Design review of the part built by this model. Coordinates are the model's own, in mm. Face numbers are marked on the shaded views. A direction names the side the tool comes from. Give positions to 0.01 mm unless a question says otherwise; leave off trailing zeros. Order: outer loops, then holes, each group sorted by start corner. A loop starts at its lowest first (then second) coordinate and runs counter-clockwise, first axis right, second up. Notation, with made-up numbers: M 1,60 L 22,60 A33 ccw 22,89 Z; hole C -12.75,38 d5. An arc over 180 degrees is marked long. Answer as a JSON object with one key per item and string values.
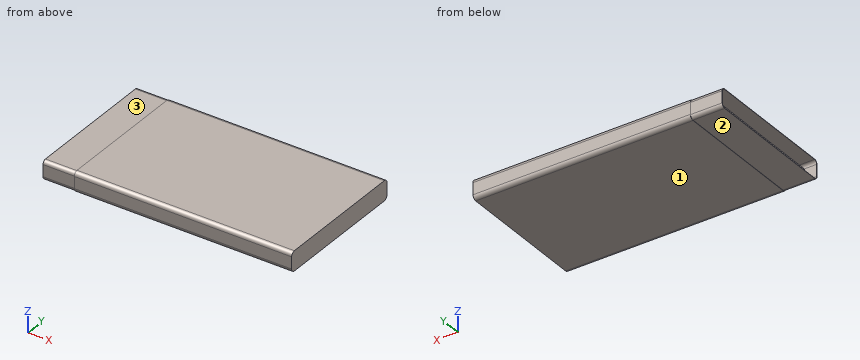
from build123d import *

# Parameters (mm, degrees)
SKETCH1_W           = 55
SKETCH1_H           = 35
BOSS_EXTRUDE1_DEPTH = 2.5
FILLET1_R           = 1
SKETCH2_W           = 5.5
SKETCH2_H           = 33
BOSS_EXTRUDE2_DEPTH = 0.8
BOSS_EXTRUDE4_DEPTH = 8


with BuildPart() as part:
    # Sketch1 → Boss-Extrude1 (new, symmetric)
    with BuildSketch(Plane.XY):
        with Locations((4, 0)):
            Rectangle(SKETCH1_W, SKETCH1_H)
    extrude(amount=BOSS_EXTRUDE1_DEPTH, both=True)

    # Fillet1
    fillet1_edges = [part.edges().sort_by_distance(p)[0] for p in [
        (4, 17.5, 2.5),
        (4, -17.5, 2.5),
        (4, 17.5, -2.5),
        (4, -17.5, -2.5),
    ]]
    fillet(fillet1_edges, radius=FILLET1_R)

    # Sketch2 → Boss-Extrude2 (add, symmetric)
    with BuildSketch(Plane.XY):
        with Locations((-26.25, 0)):
            Rectangle(SKETCH2_W, SKETCH2_H)
    extrude(amount=BOSS_EXTRUDE2_DEPTH, both=True)

    # Sketch3 → Boss-Extrude4 (add)
    with BuildSketch(Plane.ZY.offset(23.5)):
        with BuildLine():
            Line((-1.5, -17.4), (1.5, -17.4))
            ThreePointArc((1.5, -17.4), (2.136396103, -17.136396103), (2.4, -16.5))
            Line((2.4, -16.5), (2.4, 16.5))
            ThreePointArc((2.4, 16.5), (2.136396103, 17.136396103), (1.5, 17.4))
            Line((1.5, 17.4), (-1.5, 17.4))
            ThreePointArc((-1.5, 17.4), (-2.136396103, 17.136396103), (-2.4, 16.5))
            Line((-2.4, 16.5), (-2.4, -16.5))
            ThreePointArc((-2.4, -16.5), (-2.136396103, -17.136396103), (-1.5, -17.4))
        make_face()
        with BuildLine():
            Line((-1.5, -17.3), (1.5, -17.3))
            ThreePointArc((1.5, -17.3), (2.065685425, -17.065685425), (2.3, -16.5))
            Line((2.3, -16.5), (2.3, 16.5))
            ThreePointArc((2.3, 16.5), (2.065685425, 17.065685425), (1.5, 17.3))
            Line((1.5, 17.3), (-1.5, 17.3))
            ThreePointArc((-1.5, 17.3), (-2.065685425, 17.065685425), (-2.3, 16.5))
            Line((-2.3, 16.5), (-2.3, -16.5))
            ThreePointArc((-2.3, -16.5), (-2.065685425, -17.065685425), (-1.5, -17.3))
        make_face(mode=Mode.SUBTRACT)
    extrude(amount=BOSS_EXTRUDE4_DEPTH)


solid = part.part
(1) We need section B-B (y = 11). Write out the cut boundary in (x, z), plus the area to 3 significant figures.
Checked values:
{"outline": "M -31.5,-2.4 L -23.5,-2.4 L -23.5,-2.5 L 31.5,-2.5 L 31.5,2.5 L -23.5,2.5 L -23.5,2.4 L -31.5,2.4 L -31.5,2.3 L -23.5,2.3 L -23.5,0.8 L -29,0.8 L -29,-0.8 L -23.5,-0.8 L -23.5,-2.3 L -31.5,-2.3 Z", "area": "285 mm^2"}
(2) To check wall thickness, follow L1, parallel to Y at x = 18.5, z = -1.55; L2, parallel to X at y = 8.5, z = 0.7; L3, parallel to X at y = 3.5, z = -1.55. State the ranges of each line that lie inside material, in increasing order. Write a range as from..to.
Checked values:
{"L1": "y = -17.5..17.5", "L2": "x = -29..31.5", "L3": "x = -23.5..31.5"}
(3) Insertion check: pin 1 (1.6 mm diameter, centred on x = -25.5, y = -5.5, fed in from -Z); pin 2 (1.8 mm diameter, centred on y = 2.5, z = 0, fed in from -X); pin 3 (2.5 mm diameter, centred on x = -26, y = 5.5, fed in from +Z); pin 4 (1 mm diameter, centred on x = 19.5, z = -2, fed in from +Y). Each pin has a flat end and moves straight along its axis. Give the tip position at first contact, or say it passes through.
Checked values:
{"pin 1": "stops at z = -2.4", "pin 2": "stops at x = -29", "pin 3": "stops at z = 2.4", "pin 4": "stops at y = 17.5"}
(4) Tool access review of the marked faces 1, 2 and 3: name each direction out of +Z, -Z, +X, -X, +Y, -Y from which nothing blocks a thin tool from reaching the whole face with its end or side.
Checked values:
{"face 1": "-Z, +X, -X, +Y, -Y", "face 2": "-Z, -X, +Y, -Y", "face 3": "+Z, -X, +Y, -Y"}
(5) We need section A-A (x = -25.5). Write out the cut boundary in (y, z), plus the area to 3 significant figures.
Checked values:
{"outline": "M -17.4,-1.5 A0.9 ccw -16.5,-2.4 L 16.5,-2.4 A0.9 ccw 17.4,-1.5 L 17.4,1.5 A0.9 ccw 16.5,2.4 L -16.5,2.4 A0.9 ccw -17.4,1.5 Z; M -16.5,-0.8 L 16.5,-0.8 L 16.5,0.8 L -16.5,0.8 Z; hole M -17.3,-1.5 A0.8 ccw -16.5,-2.3 L 16.5,-2.3 A0.8 ccw 17.3,-1.5 L 17.3,1.5 A0.8 ccw 16.5,2.3 L -16.5,2.3 A0.8 ccw -17.3,1.5 Z", "area": "60.5 mm^2"}
